```python
from build123d import *

# Parameters (mm, degrees)
F0_W     = 83
F0_H     = 59.5
F1_DEPTH = 3
F2_R     = 2.5
F3_DEPTH = 6
F4_R     = 0.75
F5_DEPTH = 8


with BuildPart() as f1:
    # F0 (on Top) → F1 (new body)
    with BuildSketch(Plane.XY):
        with Locations((0.53559, 7.022104)):
            Rectangle(F0_W, F0_H)
    extrude(amount=F1_DEPTH)

    # F2 (on face) → F3 (join)
    with BuildSketch(Plane.XY.offset(3)):
        with Locations((-33.46441, 26.772104)):
            Circle(F2_R)
        with Locations((30.53559, 26.772104)):
            Circle(F2_R)
        with Locations((-33.46441, -17.227896)):
            Circle(F2_R)
        with Locations((30.53559, -17.227896)):
            Circle(F2_R)
    extrude(amount=F3_DEPTH)

    # F4 (on face) → F5 (join)
    with BuildSketch(Plane.XY.offset(3)):
        with Locations((-33.46441, 26.772104)):
            Circle(F4_R)
        with Locations((30.53559, 26.772104)):
            Circle(F4_R)
        with Locations((30.53559, -17.227896)):
            Circle(F4_R)
        with Locations((-33.46441, -17.227896)):
            Circle(F4_R)
    extrude(amount=F5_DEPTH)


solid = f1.part
```
The listing builds one solid part. Answer for the finished solid, in the listing's coordinates (mm). A direction names the side the tool comes from. Coordinates: 2 decimals unless noted, no trailing zeros. Order: outer loops, then holes, each group sorted by start corner. A loop starts at its lowest first (then second) coordinate and runs counter-clockwise, first axis right, second up. Notation, with made-up numbers: M 34.25,-29 L 64.25,-29 A21 cw 64.25,-15 Z; hole C 14.5,10.5 d7. An arc over 180 degrees is marked long. Answer as a JSON object with one key per item and string values. Group by question number.
1. Section A-A on y = -13 is taken. Write down the section's boundary in (x, z).
2. Section B-B on x = -11.5 is taken. Write down the section's boundary in (y, z).
3. Section C-C on z = 8 is taken. Write down the section's boundary in (x, y).
4. Straight lines are drawn through the part: line 1 (Z direction, x = 21.5, y = 14); line 2 (Z direction, x = -33, y = 28); line 3 (X direction, y = -16, z = 4.25). For each, find the intervals that lie inside material, in ascending order.
5. A tool of negligible diameter and unlimited length cuts with its end or side. For faces 1 (the flat face through (30, -18, 9)), 2 (the flat face through (0, -22.728, 1)), from which of +Z, -Z, +X, -X, +Y, -Y can it reach the whole face along a straight path? Write none if from no direction.
6. Flat-ended cylindrical pins translate along their axes: P1, Ø3, axis at x = 20.5, y = 4, coming from the +Z side; P2, Ø3, axis at y = 30, z = 8.5, coming from the -X side. Find the tip coordinate at first contact, or state that the pin passes through.
7. Determine the mould class of faces 3 (the flat face through (0, 36.772, 1)), 4 (the cylindrical face through (-33.79, 29.25, 5.96)), 5 (the flat face through (-40.964, 7, 1)) for opening direction Y: released by +Y, released by -Y, zero draft, split by the parting line, or undercut.
Values follow:
{
 "1": {"outline": "M -40.96,0 L 42.04,0 L 42.04,3 L -40.96,3 Z"},
 "2": {"outline": "M -22.73,0 L 36.77,0 L 36.77,3 L -22.73,3 Z"},
 "3": {"outline": "C -33.46,-17.23 d5; C -33.46,26.77 d5; C 30.54,-17.23 d5; C 30.54,26.77 d5"},
 "4": {"line 1": "0 to 3", "line 2": "0 to 9", "line 3": "-35.64 to -31.29, 28.36 to 32.71"},
 "5": {"face 1": "+Z", "face 2": "+Z, -Z, +X, -X, -Y"},
 "6": {"P1": "z = 3", "P2": "x = -35.27"},
 "7": {"face 3": "released by +Y", "face 4": "undercut", "face 5": "zero draft"}
}
